Input: dimensioned drawing with shaded views. Units: mm. Origin: part minimum x, y, z. Round coordinates to 2 decimals unless told otherwise and drop trailing zeros. Write each loop counter-clockwise with the first axis right and the second up, starting at its lowest first coordinate (ties: lowest second). Pieces come first, ordered by that corner, then holes. Notation, with made-up numbers: (19.25, 84) -> (34.25, 84) arc R23 ccw to (34.25, 110) -> close; hole circle Ø6 at (10, -4.5). An arc over 180 degrees is marked (long way). Use one line per item in the form item = value. Start each with the question number.
1. Line query: L1, parallel to Z at x = 39, y = 0.7; L2, parallel to Z at x = 23, y = 1.8; L3, parallel to X at y = 1, z = 39.5. Output: solid intervals per line, ascending.
2. Pin query (flat end, axial travel): pin 1 Ø0.6 at (x, y) = (20.5, 1) entering from -Z; pin 2 Ø0.9 at (x, y) = (36, 1) entering from -Z; pin 3 Ø1.5 at (y, z) = (1.5, 11) entering from -X. Return the tip coordinate at first contact, or that it passes through.
3. Cut plane A-A, the plane z = 40. Return the cut outline in (x, y).
4. Cut plane C-C, the plane x = 3.5. Return the cut outline in (y, z), plus the area to 3 significant figures.
5. Cut plane B-B, the plane z = 13. Return the cut outline in (x, y).
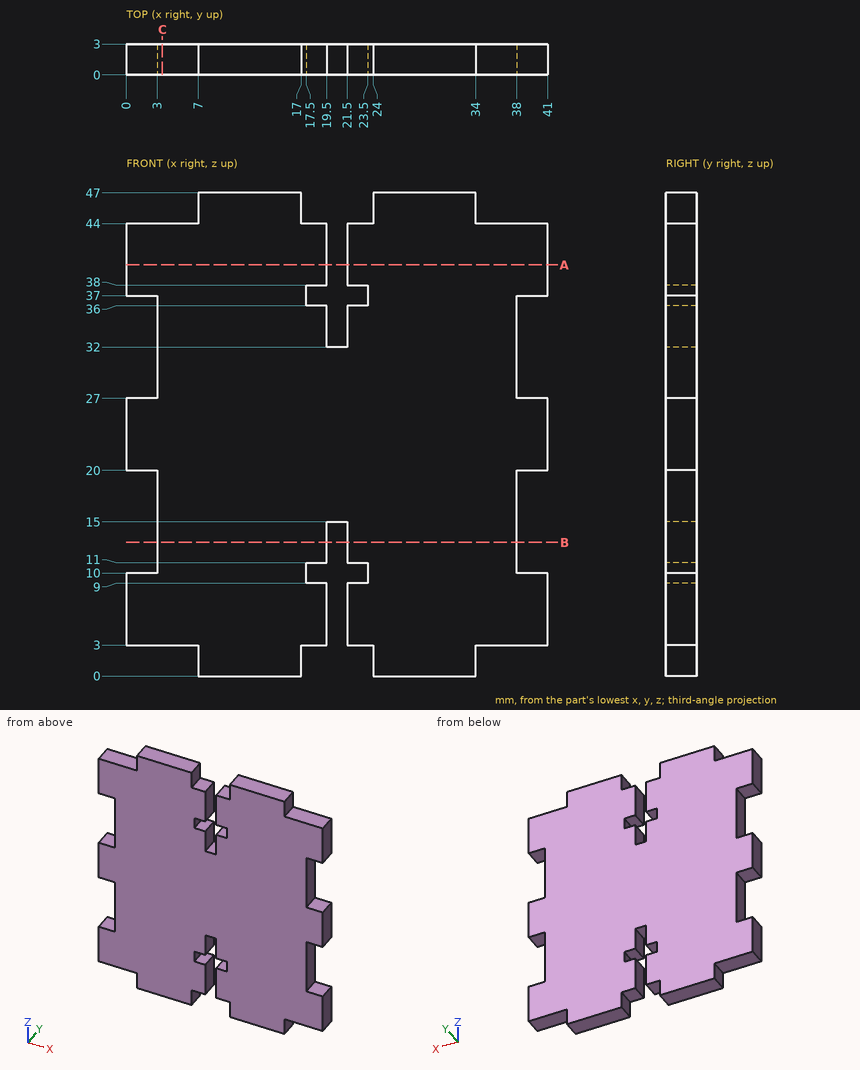
Outcome:
q1.L1 = 3 to 10, 20 to 27, 37 to 44
q1.L2 = 3 to 9, 11 to 36, 38 to 44
q1.L3 = 0 to 19.5, 21.5 to 41
q2.pin_1 = 15
q2.pin_2 = 3
q2.pin_3 = 3
q3.outline = (0, 0) -> (19.5, 0) -> (19.5, 3) -> (0, 3) -> close; (21.5, 0) -> (41, 0) -> (41, 3) -> (21.5, 3) -> close
q4.outline = (0, 3) -> (3, 3) -> (3, 44) -> (0, 44) -> close
q4.area = 123 mm^2
q5.outline = (3, 0) -> (19.5, 0) -> (19.5, 3) -> (3, 3) -> close; (21.5, 0) -> (38, 0) -> (38, 3) -> (21.5, 3) -> close
